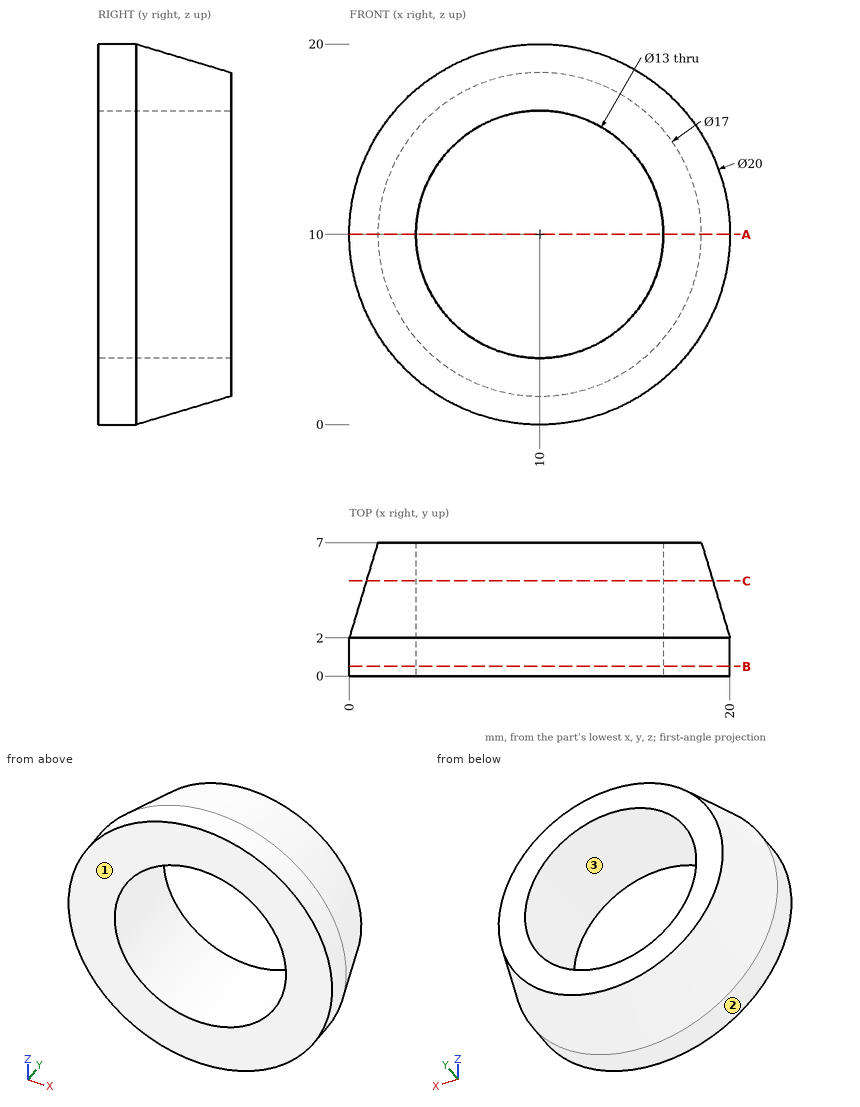
Drawing for the job (mm, zero at the part's lowest x, y, z). Give positions to 0.01 mm unless a question says otherwise; leave off trailing zeros. Write each loop counter-clockwise with the first axis right and the second up, starting at its lowest first coordinate (ties: lowest second). Pieces come first, ordered by that corner, then holes. Notation, with made-up numbers: (88.25, 31) -> (109.25, 31) arc R29 ccw to (109.25, 66) -> close; hole circle Ø7 at (-7, -7.5). An arc over 180 degrees is marked (long way). Put each result on its own line as item: value. Start each with the question number.
Item 1: Cut at A-A (z = 10). List the corners of the cut face in (x, y).
Item 2: Cut at C-C (y = 5). List the corners of the cut face in (x, z), then the cut area to 3 significant figures.
Item 3: Cut at B-B (y = 0.5). List the corners of the cut face in (x, z), then the cut area to 3 significant figures.
Item 4: Pull direction X, two halves, no side cores. Call the marked faces 1, 2 and 3: pulls with the +X half, pulls with the -X half, needs draft (parallel to the pull), parting line crosses it, or undercut.
Item 5: Pin check, flat tip, straight feed: pin 1 Ø8 at (x, z) = (10, 10) entering from +Y. Stop position of the tip, or through.
Item 6: Wall check: L1, parallel to X at y = 4, z = 5; L2, parallel to Z at x = 6.75, y = 3.5; L3, parallel to X at y = 5.25, z = 10 (3 decimals). Give the ranges that are in metal, low to high. Write a range as [from, to].
Answer list:
1. outline: (0, 0) -> (3.5, 0) -> (3.5, 7) -> (1.5, 7) -> (0, 2) -> close; (16.5, 0) -> (20, 0) -> (20, 2) -> (18.5, 7) -> (16.5, 7) -> close
2. outline: circle Ø18.2 at (10, 10); hole circle Ø13 at (10, 10)
2. area: 127 mm2
3. outline: circle Ø20 at (10, 10); hole circle Ø13 at (10, 10)
3. area: 181 mm2
4. face 1: needs draft
4. face 2: parting line crosses it
4. face 3: undercut
5. pin 1: passes through
6. L1: x = [2.04, 5.85], [14.15, 17.96]
6. L2: z = [1.02, 4.37], [15.63, 18.98]
6. L3: x = [0.975, 3.5], [16.5, 19.025]
